Could you check a few things on this drawing? It's one solid part, dimensions in mm from its lowest x, y, z. A direction names the side the tool comes from. Give positions to 0.01 mm unless a question says otherwise; leave off trailing zeros. Loops run counter-clockwise (first coordinate to the right, second up) from the corner with the lowest first, then second, coordinate; pieces in that order, holes last.
Q1. I'm going to push flat-ended pins straight in: P1, Ø6, axis at y = 14, z = 30.5, coming from the -X side; P2, Ø2.5, axis at x = 34, z = 24, coming from the +Y side; P3, Ø1, axis at x = 40.5, y = 7.5, coming from the -Z side; P4, Ø1.5, axis at x = 21, z = 6.5, coming from the +Y side. Where does each tip first touch, or does it pass through?
Q2. Suppose I cut it at C-C (y = 5.5). List the corners of the cut face in (x, z) for me.
Q3. I need wall thicknesses on probe 1 along X at (y, z) = (10.5, 24); probe 2 along Z at (x, y) = (22.5, 10); probe 3 along Z at (x, y) = (22, 14). Which ranges of each line are inside material? Lowest first, please.
Q4. Suppose I cut it at D-D (x = 24). List the corners of the cut face in (y, z) for me.
Q5. Thinking about a two-plate mould opening in Z: for the marked faces 3, 4 and 5, which applies, pulls with the +Z half, pulls with the -Z half, needs draft (parallel to the pull), parting line crosses it, or undercut?
Q6. Suppose I cut it at B-B (x = 34). List the corners of the cut face in (y, z) for me, and give its area (3 significant figures).
Q7. Suppose I cut it at A-A (z = 24). List the corners of the cut face in (x, y) for me.
Q8. For the marked faces 1 and 2, which set-ups out of +Z, -Z, +X, -X, +Y, -Y let a thin tool reach every point of the face, with its end or its side?
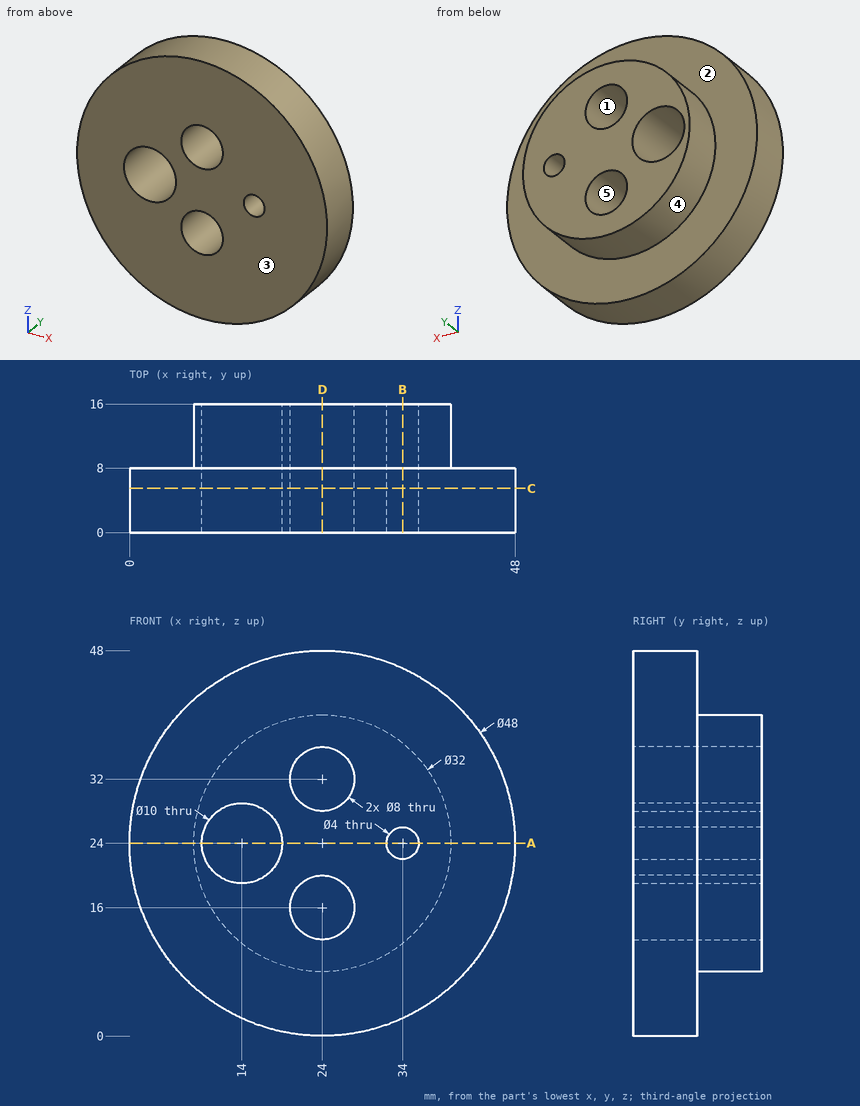
Solutions:
1. P1: stops at x = 8.39
1. P2: passes through
1. P3: stops at z = 6.11
1. P4: stops at y = 8
2. outline: circle Ø48 at (24, 24); hole circle Ø10 at (14, 24); hole circle Ø8 at (24, 16); hole circle Ø8 at (24, 32); hole circle Ø4 at (34, 24)
3. probe 1: x = 8 to 9, 19 to 32, 36 to 40
3. probe 2: z = 8.07 to 12.29, 19.71 to 28.29, 35.71 to 39.93
3. probe 3: z = 8.13 to 12.54, 19.46 to 28.54, 35.46 to 39.87
4. outline: (0, 0) - (8, 0) - (8, 8) - (16, 8) - (16, 12) - (0, 12) - close; (0, 20) - (16, 20) - (16, 28) - (0, 28) - close; (0, 36) - (16, 36) - (16, 40) - (8, 40) - (8, 48) - (0, 48) - close
5. face 3: needs draft
5. face 4: parting line crosses it
5. face 5: undercut
6. outline: (0, 2.18) - (8, 2.18) - (8, 11.51) - (16, 11.51) - (16, 22) - (0, 22) - close; (0, 26) - (16, 26) - (16, 36.49) - (8, 36.49) - (8, 45.82) - (0, 45.82) - close
6. area: 485 mm2
7. outline: (0, 0) - (9, 0) - (9, 16) - (8, 16) - (8, 8) - (0, 8) - close; (19, 0) - (32, 0) - (32, 16) - (19, 16) - close; (36, 0) - (48, 0) - (48, 8) - (40, 8) - (40, 16) - (36, 16) - close
8. face 1: +Y, -Y
8. face 2: +Y
